Can you work these out from the model? Positions are in its coordinate system, mm. A direction names the side the tool comes from. Give positions to 0.01 mm unless a question says otherwise; leave off trailing zeros. Write each loop counter-clockwise with the first axis right and the second up, starting at its lowest first coordinate (ties: lowest second). Pieces come first, ordered by that corner, then holes.
1. Suppose I cut it at A-A (z = 4.25). Please give me the cut outline in (x, y), and give its area (3 significant figures).
2. Thinking about a two-plate mould opening in Y: for faces 3 (the cylindrical face through (-1.73, -7.81, 5.04)), 4 (the flat face through (2.5, 2.8, 0)), 5 (the cylindrical face through (-6, 0, 4)), 6 (the cylindrical face through (9.54, -3, 3.99)), which applies, pulls with the +Y half, pulls with the -Y half, needs draft (parallel to the pull), parting line crosses it, or undercut?
3. If I drill on probe 1 along Y at (x, z) = (0, 4.75); probe 2 along Z at (x, y) = (4, -10.25); probe 3 along Y at (x, z) = (2.75, 4), over which ranges is the centre line in solid material (lowest first)?
4. On a 3-axis mill with a long thin cutter (end or side, diameter ignored), from which of +Z, -Z, +X, -X, +Y, -Y can I reach the whole of each face in a straight line? I mean faces 1 (the cylindrical face through (-0.867, 3.905, 3.873)), 2 (the cylindrical face through (-11.99, -0.53, 7.75)). Say none if no direction works.
5. Suppose I cut it at B-B (z = 7). Please give me the cut outline in (x, y), and give its area (3 significant figures).
6. I'm going to push flat-ended pins straight in: pin 1 (1.5 mm diameter, centred on x = -1, z = 6, fed in from +Y); pin 2 (3.5 mm diameter, centred on x = 0.5, y = -2, fed in from +Z); pin 3 (2.5 mm diameter, centred on x = -0.5, y = -2, fed in from +Z); pin 4 (10.5 mm diameter, centred on x = 0, y = 0, fed in from +Z). Where does each tip first touch, or does it pass through?
Autodesk Inventor part; units mm, degrees
ref_plane "YZ Plane" through (0, 0, 0) normal (1, 0, 0) x (0, 1, 0)
ref_plane "XZ Plane" through (0, 0, 0) normal (0, 1, 0) x (-1, 0, 0)
ref_plane "XY Plane" through (0, 0, 0) normal (0, 0, 1) x (1, 0, 0)
sketch "Sketch1" plane through (0, 0, 0) normal (0, 0, 1) x (1, 0, 0)
  circle A0 centre (0, 0) radius 12
  dimension "d0" = 24
extrude "Extrusion1" add sketch "Sketch1" along normal blind 2
sketch "Sketch2" plane through (0, 0, 2) normal (0, 0, 1) x (1, 0, 0)
  circle A0 centre (0, 0) radius 12
  circle A1 centre (0, 0) radius 10
  dimension "d4" = 20
extrude "Extrusion2" add sketch "Sketch2" along normal blind 4 contours A1
sketch "Sketch3" plane through (0, 0, 6) normal (0, 0, 1) x (1, 0, 0)
  circle A0 centre (0, 0) radius 10
  circle A1 centre (0, 0) radius 12
  dimension "d26" = 24
extrude "Extrusion3" add sketch "Sketch3" along normal blind 2 contours A0 | A1
fillet "Fillet1" radius 1.5 4 edges at (-12, 0, 6) (-10, 0, 6) (-12, 0, 2) (-10, 0, 2)
sketch "Sketch7" plane through (0, 0, 8) normal (0, 0, 1) x (1, 0, 0)
  circle A0 centre (0, 0) radius 12
  circle A1 centre (0, 0) radius 8
  dimension "d29" = 16
extrude "Extrusion7" cut sketch "Sketch7" against normal blind 6 contours A1
sketch "Sketch8" plane through (0, 0, 2) normal (0, 0, 1) x (1, 0, 0)
  circle A0 centre (0, 0) radius 8
  circle A1 centre (0, 0) radius 3.5
  dimension "d36" = 7
extrude "Extrusion8" cut sketch "Sketch8" against normal blind 8 contours A1
sketch "Sketch9" plane through (0, 0, 2) normal (0, 0, 1) x (1, 0, 0)
  circle A0 centre (0, 0) radius 8
  circle A1 centre (0, 0) radius 4
  circle A2 centre (0, 0) radius 6
  dimension "d40" = 12
  dimension "d41" = 8
extrude "Extrusion9" add sketch "Sketch9" along normal blind 3.8 contours A2
properties part number "guidance wheel"
Checks:
1. outline: circle Ø20 at (0, 0); circle Ø12 at (0, 0); hole circle Ø16 at (0, 0); hole circle Ø8 at (0, 0)
1. area: 176 mm2
2. face 3: undercut
2. face 4: needs draft
2. face 5: undercut
2. face 6: parting line crosses it
3. probe 1: y = -10 to -8, -6 to -4, 4 to 6, 8 to 10
3. probe 2: z = 0 to 1.91, 6.09 to 8
3. probe 3: y = -9.61 to -7.51, -5.33 to -2.9, 2.9 to 5.33, 7.51 to 9.61
4. face 1: +Z
4. face 2: +Z, -Z
5. outline: circle Ø23.83 at (0, 0); hole circle Ø16 at (0, 0)
5. area: 245 mm2
6. pin 1: stops at y = 11.76
6. pin 2: stops at z = 2
6. pin 3: passes through
6. pin 4: stops at z = 5.8
